Geometry: final body of the model. Coordinates: model frame, mm. Face numbers are marked on the shaded views. A direction names the side the tool comes from. Give positions to 0.01 mm unless a question says otherwise; leave off trailing zeros. Write each loop counter-clockwise with the first axis right and the second up, starting at its lowest first coordinate (ties: lowest second). Pieces come first, ordered by that corner, then holes.
```python
from build123d import *

# Parameters (mm, degrees)
F1_DEPTH = 63.5
F2_DEPTH = 25.4
F4_DEPTH = 7.9375
F5_R     = 5.08


with BuildPart() as f1:
    # F0 (on Front) → F1 (new body, symmetric)
    with BuildSketch(Plane.XZ):
        Polygon((41.275, -9.525), (41.275, 9.525), (22.225, 9.525), (-41.275, 9.525), (-41.275, -9.525), align=None)
    extrude(amount=F1_DEPTH, both=True)

    # F0 (on Front) → F2 (join, symmetric)
    with BuildSketch(Plane.XZ):
        with BuildLine():
            Line((22.225, 9.525), (41.275, 9.525))
            Line((41.275, 9.525), (41.275, 27.0002))
            ThreePointArc((41.275, 27.0002), (45.92468, 38.22552), (57.15, 42.8752))
            Line((57.15, 42.8752), (60.325, 42.8752))
            Line((60.325, 42.8752), (60.325, 61.9252))
            Line((60.325, 61.9252), (57.15, 61.9252))
            ThreePointArc((57.15, 61.9252), (32.454296, 51.695904), (22.225, 27.0002))
            Line((22.225, 27.0002), (22.225, 9.525))
        make_face()
        Polygon((60.325, 61.9252), (60.325, 42.8752), (85.725, 42.8752), (85.725, 51.485013), (85.725, 61.9252), align=None)
    extrude(amount=F2_DEPTH, both=True)

    # F0 (on Front) → F3 (revolve)
    with BuildSketch(Plane.XZ):
        Polygon((85.725, 51.485013), (85.725, 42.8752), (85.725, 37.197513), (111.125, 37.197513), (111.125, 65.772513), (85.725, 65.772513), (85.725, 61.9252), align=None)
    revolve(axis=Axis((85.725, 0, 56.705107), (0, 0, -1)))

    # F0 (on Front) → F4 (join, symmetric)
    with BuildSketch(Plane.XZ):
        with BuildLine():
            Line((-41.275, 9.525), (22.225, 9.525))
            Line((22.225, 9.525), (22.225, 27.0002))
            ThreePointArc((22.225, 27.0002), (32.454296, 51.695904), (57.15, 61.9252))
            add(Edge.make_bspline(
                [(57.15, 61.9252), (9.904783, 63.30175), (-40.170714, 38.131271), (-41.275, 9.525)],
                knots=[0, 0, 0, 0, 111.504536, 111.504536, 111.504536, 111.504536], degree=3))
        make_face()
    extrude(amount=F4_DEPTH, both=True)

    # F5
    f5_edges = [f1.edges().sort_by_distance(p)[0] for p in [
        (41.275, 63.5, 0),
        (-41.275, 63.5, 0),
        (-41.275, -63.5, 0),
        (41.275, -63.5, 0),
    ]]
    fillet(f5_edges, radius=F5_R)


solid = f1.part
```
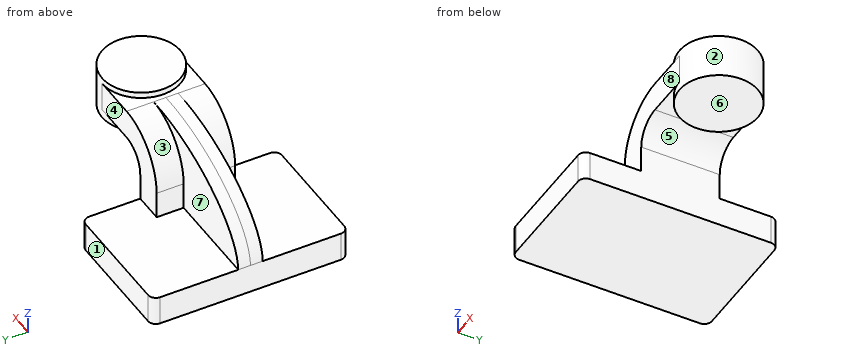
Item 1: Line query: L1, parallel to Z at x = 24, y = 43.5 (3 decimals); L2, parallel to Z at x = 87, y = -13; L3, parallel to X at y = 18.5, z = -3 (3 decimals). Output: solid intervals per line, ascending.
Found:
L1: z = -9.525 to 9.525
L2: z = 37.2 to 65.77
L3: x = -41.275 to 41.275
Item 2: Reachability of the marked faces 4, 5, 6, 7 and 8 from +Z, -Z, +X, -X, +Y, -Y: full face, straight path, thin tool, end or side. Return the list, or none.
Found:
face 4: +Z, +X, -X, +Y
face 5: -Z, +Y, -Y
face 6: -Z, +X, +Y, -Y
face 7: +Z, -X, +Y
face 8: +Z, +X, -X, -Y
Item 3: Section A-A, the plane y = -48.5. Return the cut outline in (x, z) (3 decimals), plus the area to 3 significant figures.
Found:
outline: (-41.275, -9.525) - (41.275, -9.525) - (41.275, 9.525) - (-41.275, 9.525) - close
area: 1,570 mm2
Item 4: Pull-direction query (X, two-part tool) for the marked faces 1, 2 and 3; classes: +X half, -X half, draft (parallel to the pull), parting line (faces both ways), or undercut.
Found:
face 1: draft
face 2: undercut
face 3: -X half
Item 5: Pin query (flat end, axial travel): pin 1 Ø5 at (x, y) = (70.5, -11.5) entering from -Z; pin 2 Ø4 at (y, z) = (-6, 35.5) entering from +X; pin 3 Ø10 at (y, z) = (19, 20) entering from +X (3 decimals). Return the tip coordinate at first contact, or that it passes through.
Found:
pin 1: stops at z = 37.2
pin 2: stops at x = 110.64
pin 3: stops at x = 41.275
